Part model, mm, in its own coordinate system. A direction names the side the tool comes from. Round coordinates to 2 decimals unless told otherwise and drop trailing zeros. Loops run counter-clockwise (first coordinate to the right, second up) from the corner with the lowest first, then second, coordinate; pieces in that order, holes last.
Autodesk Inventor part; units mm, degrees
ref_plane "YZ Plane" through (0, 0, 0) normal (1, 0, 0) x (0, 1, 0)
ref_plane "XZ Plane" through (0, 0, 0) normal (0, 1, 0) x (-1, 0, 0)
ref_plane "XY Plane" through (0, 0, 0) normal (0, 0, 1) x (1, 0, 0)
sketch "Sketch1" plane through (0, 0, 0) normal (0, 1, 0) x (-1, 0, 0)
  line L0 (30.4, 18.2) -> (-30.4, 18.2)
  line L1 (-30.4, 18.2) -> (-30.4, -18.2)
  line L2 (-30.4, -18.2) -> (30.4, -18.2)
  line L3 (30.4, -18.2) -> (30.4, 18.2)
  point P0 (0, 0)
  dimension "d0" = 60.8
  dimension "d1" = 36.4
extrude "Extrusion1" add sketch "Sketch1" along normal blind 5
sketch "Sketch2" plane through (0, 5, 0) normal (0, 1, 0) x (1, 0, 0)
  line L0 (30.4, 18.2) -> (-30.4, 18.2)
  line L1 (-30.4, 18.2) -> (-0.4, 18.2)
  line L2 (-0.4, 18.2) -> (-0.4, 13.2)
  line L3 (-0.4, 13.2) -> (-30.4, 13.2)
  line L4 (-30.4, 13.2) -> (-30.4, 18.2)
  line L5 (30.4, -18.2) -> (30.4, 18.2)
  line L6 (30.4, -18.2) -> (0.4, -18.2)
  line L7 (0.4, -18.2) -> (0.4, -13.2)
  line L8 (0.4, -13.2) -> (30.4, -13.2)
  line L9 (30.4, -13.2) -> (30.4, -18.2)
  point P0 (0, 0)
  dimension "d4" = 30
  dimension "d5" = 5
  dimension "d6" = 30
  dimension "d7" = 5
extrude "Extrusion2" add sketch "Sketch2" along normal blind 24.4
sketch "Sketch3" plane through (0, 5, 0) normal (0, 1, 0) x (1, 0, 0)
  circle A0 centre (12.7, 0) radius 4.325
  circle A1 centre (-12.7, 0) radius 4.325
  point P0 (0, 0)
  dimension "d10" = 8.65
  dimension "d11" = 8.65
extrude "Extrusion3" add sketch "Sketch3" along normal blind 5
sketch "Sketch4" plane through (-12.7, 10, 0) normal (0, 1, 0) x (1, 0, 0)
  circle A0 centre (0, 0) radius 2
  circle A1 centre (25.4, 0) radius 4.325
  circle A2 centre (25.4, 0) radius 2
  point P0 (12.7, 0)
  dimension "d14" = 4
  dimension "d15" = 4
extrude "Extrusion4" cut sketch "Sketch4" against normal blind 15 contours A0 | A2
sketch "Sketch5" plane through (0, 0, 0) normal (0, -1, 0) x (1, 0, 0)
  circle A0 centre (12.7, 0) radius 2
  circle A1 centre (12.7, 0) radius 3
  circle A2 centre (-12.7, 0) radius 2
  circle A3 centre (-12.7, 0) radius 3
  point P0 (0, 0)
  dimension "d18" = 6
  dimension "d19" = 6
extrude "Extrusion5" cut sketch "Sketch5" against normal blind 3 contours A0 | A1 | A2 | A3
chamfer "Chamfer1" distance 1.5 angle 45 2 edges at (8.375, 10, 0) (-17.025, 10, 0)
sketch "Sketch6" plane through (0, 0, 0) normal (0, -1, 0) x (1, 0, 0)
  line L0 (-28.4, -18.2) -> (28.4, -18.2)
  line L1 (30.4, 18.2) -> (-4, 18.2)
  line L2 (-4, 18.2) -> (-4, -18.2)
  line L3 (-4, -18.2) -> (30.4, -18.2)
  line L4 (30.4, -18.2) -> (30.4, 18.2)
  line L5 (1.5875, 26.9875) -> (-34.925, 26.9875)
  line L6 (-34.925, 26.9875) -> (-34.925, -36.5125)
  line L7 (-34.925, -36.5125) -> (1.5875, -36.5125)
  line L8 (1.5875, -36.5125) -> (1.5875, 26.9875)
  point P0 (0, 0)
  point P1 (1.5875, -18.2)
  point P2 (1.5875, 18.2)
  dimension "d26" = 34.4
extrude "Extrusion6" cut sketch "Sketch6" against normal blind 50 contours L0 L8 L7 L6 L5 L1 L2
sketch "Sketch7" plane through (0, 29.4, 0) normal (0, 1, 0) x (1, 0, 0)
  line L0 (30.4, 18.2) -> (-4, 18.2)
  line L1 (30.4, -13.2) -> (30.4, 18.2)
  line L2 (-4, 18.2) -> (30.4, 18.2)
  line L3 (30.4, 18.2) -> (30.4, 13.2)
  line L4 (30.4, 13.2) -> (-4, 13.2)
  line L5 (-4, 13.2) -> (-4, 18.2)
  line L6 (-4, -18.2) -> (30.4, -18.2)
  line L7 (-4, 13.2) -> (-4, -18.2)
  line L8 (30.4, -18.2) -> (-4, -18.2)
  line L9 (-4, -18.2) -> (-4, -13.2)
  line L10 (-4, -13.2) -> (30.4, -13.2)
  line L11 (30.4, -13.2) -> (30.4, -18.2)
  point P0 (0, 0)
  dimension "d29" = 5
  dimension "d30" = 5
extrude "Extrusion7" add sketch "Sketch7" against normal blind 27 contours L1 L4 L5 L0 | L11 L6 L7 L10
sketch "Sketch8" plane through (0, 29.4, 0) normal (0, 1, 0) x (1, 0, 0)
  line L0 (-4, -18.2) -> (-4, 18.2)
  line L1 (30.4, 13.2) -> (-4, 13.2)
  line L2 (-4, 18.2) -> (30.4, 18.2)
  line L3 (30.4, 18.2) -> (30.4, 13.2)
  line L4 (30.4, 13.2) -> (-4, 13.2)
  line L5 (-4, 13.2) -> (-4, 18.2)
  line L6 (-4, -18.2) -> (30.4, -18.2)
  line L7 (-4, -13.2) -> (30.4, -13.2)
  line L8 (30.4, -18.2) -> (-4, -18.2)
  line L9 (-4, -18.2) -> (-4, -13.2)
  line L10 (-4, -13.2) -> (30.4, -13.2)
  line L11 (30.4, -13.2) -> (30.4, -18.2)
  point P0 (0, 0)
extrude "Extrusion8" cut sketch "Sketch8" against normal blind 2
fillet "Fillet2" radius 2 8 edges at (30.4, 13.7, -18.2) (-4, 13.7, 18.2) (-4, 13.7, -18.2) (30.4, 13.7, 18.2) (30.4, 0, 0) (-4, 0, 0) (13.2, 0, 18.2) (13.2, 0, -18.2)
properties part number "centerMount"
1) Slice it at B-B, the plane z = 0. Give the cut face in (x, y) (3 decimals).
Values:
outline: (-4, 2) arc R2 ccw to (-2, 0) - (9.7, 0) - (9.7, 3) - (10.7, 3) - (10.7, 10) - (9.875, 10) - (8.375, 8.5) - (8.375, 5) - (-4, 5) - close; (14.7, 3) - (15.7, 3) - (15.7, 0) - (28.4, 0) arc R2 ccw to (30.4, 2) - (30.4, 5) - (17.025, 5) - (17.025, 8.5) - (15.525, 10) - (14.7, 10) - close
2) Slice it at D-D, the plane y = 20. Give the cut face in (x, z), then the cut area to 3 significant figures.
Values:
outline: (-4, -16.2) arc R2 ccw to (-2, -18.2) - (28.4, -18.2) arc R2 ccw to (30.4, -16.2) - (30.4, -13.2) - (-4, -13.2) - close; (-4, 13.2) - (30.4, 13.2) - (30.4, 16.2) arc R2 ccw to (28.4, 18.2) - (-2, 18.2) arc R2 ccw to (-4, 16.2) - close
area: 341 mm2
3) Mould opens along X. For faces 3 (the face through (13.41, 0.6, 17.63)), 4 (the face through (-3.43, 14.52, -17.6)), 5 (the face through (29.83, 14.88, -17.6)), 6 (the face through (15.47, 1.48, -1.15)) say: released by +X, released by -X, zero draft, split by the parting line, or undercut.
Values:
face 3: zero draft
face 4: released by -X
face 5: released by +X
face 6: undercut
4) Drop flat-ended pins along their axis: pin 1 Ø1.8 at (x, z) = (12, 0) entering from -Y; pin 2 Ø4.5 at (x, z) = (13, -1) entering from +Y; pin 3 Ø6 at (x, z) = (1, 8.5) entering from +Y. Give the stop position or say it passes through.
Values:
pin 1: passes through
pin 2: stops at y = 10
pin 3: stops at y = 5
5) Wall check: line 1 along Z through (x, y) = (12.7, 7.25) (3 decimals); line 2 along X through (y, z) = (7.5, 0) (3 decimals); line 3 along Z through (x, y) = (10, 13.5). Give the ranges that are in metal, low to high.
Values:
line 1: z = -18.2 to -13.2, -4.325 to -2, 2 to 4.325, 13.2 to 18.2
line 2: x = 8.375 to 10.7, 14.7 to 17.025
line 3: z = -18.2 to -13.2, 13.2 to 18.2
6) Slice it at C-C, the plane x = 12.7. Give the cut face in (y, z) (3 decimals).
Values:
outline: (0, -16.2) arc R2 ccw to (2, -18.2) - (27.4, -18.2) - (27.4, -13.2) - (5, -13.2) - (5, -4.325) - (8.5, -4.325) - (10, -2.825) - (10, -2) - (3, -2) - (3, -3) - (0, -3) - close; (0, 3) - (3, 3) - (3, 2) - (10, 2) - (10, 2.825) - (8.5, 4.325) - (5, 4.325) - (5, 13.2) - (27.4, 13.2) - (27.4, 18.2) - (2, 18.2) arc R2 ccw to (0, 16.2) - close
7) Tool access for faces 1 (the face through (14, 10, 2)), 2 (the face through (17, 0, 0)): list every direction of +Z, -Z, +X, -X, +Y, -Y with a clear straight run to the whole face (end or side of a thin tool).
Values:
face 1: +X, -X, +Y
face 2: +Z, -Z, +X, -X, -Y
8) Slice it at A-A, the plane y = 5.75. Give the cut face in (x, z) (3 decimals).
Values:
outline: (-4, -16.2) arc R2 ccw to (-2, -18.2) - (28.4, -18.2) arc R2 ccw to (30.4, -16.2) - (30.4, -13.2) - (-4, -13.2) - close; (-4, 13.2) - (30.4, 13.2) - (30.4, 16.2) arc R2 ccw to (28.4, 18.2) - (-2, 18.2) arc R2 ccw to (-4, 16.2) - close; circle Ø8.65 at (12.7, 0); hole circle Ø4 at (12.7, 0)
